Source: CAD feature listing. Evaluate the final solid. Frame: model axes, mm. Give positions to 0.01 mm unless a question says otherwise; leave off trailing zeros. Write each loop counter-clockwise with the first axis right and the second up, starting at its lowest first coordinate (ties: lowest second). Pieces come first, ordered by that corner, then holes. Notation, with made-up numbers: M -16,0 L 17,0 A25 cw 17,16 Z; hole C 37,-6 d9. An arc over 180 degrees is marked long. Use CSV: the item, a comma, the result in double quotes. Start each with the question number.
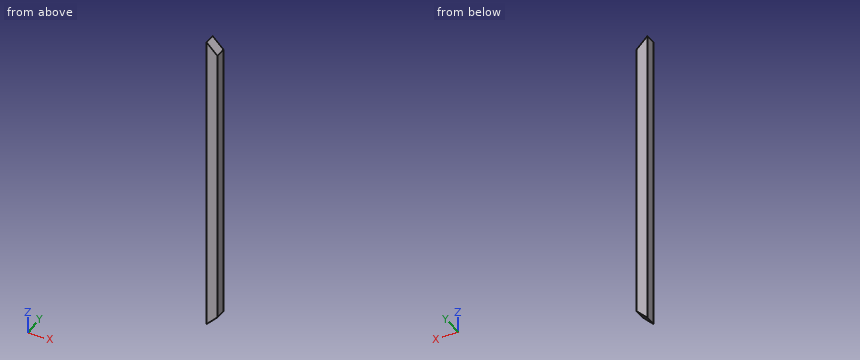
from build123d import *

# Parameters (mm, degrees)
F0_W     = 38.1
F0_H     = 38.1
F1_DEPTH = 1066.8
F3_DEPTH = 38.1
F4_DEPTH = 38.1


with BuildPart() as f1:
    # F0 (on Top) → F1 (new body)
    with BuildSketch(Plane.XY):
        Rectangle(F0_W, F0_H)
    extrude(amount=F1_DEPTH)

    # F2 (on face) → F3 (cut)
    with BuildSketch(Plane.XZ.offset(19.05)):
        Polygon((19.05, 1066.8), (-19.05, 1066.8), (19.05, 1028.7), align=None)
    extrude(amount=-F3_DEPTH, mode=Mode.SUBTRACT)

    # F2 (on face) → F4 (cut)
    with BuildSketch(Plane.XZ.offset(19.05)):
        Polygon((19.05, 38.1), (-19.05, 0), (19.05, 0), align=None)
    extrude(amount=-F4_DEPTH, mode=Mode.SUBTRACT)


solid = f1.part
Item 1: Material intervals for probe 1 along Z at (x, y) = (12, 7.5); probe 2 along Z at (x, y) = (-10, 10), sorted ascending.
Item 2: Section B-B (y = 1). Return the cut outline in (x, z), plus the area to 3 significant figures.
Item 3: Contact query for flat-ended pins moving along their axis: pin 1 Ø2 at (x, y) = (5.5, -12) entering from -Z; pin 2 Ø1.5 at (x, y) = (12.5, 12.5) entering from +Z; pin 3 Ø1.5 at (x, y) = (-1.5, -11.5) entering from -Z. Output: stop coordinate, or through.
Item 4: Section A-A (x = 3). Return the cut outline in (y, z).
Output values:
1,probe 1,"z = 31.05 to 1035.75"
1,probe 2,"z = 9.05 to 1057.75"
2,outline,"M -19.05,0 L 19.05,38.1 L 19.05,1028.7 L -19.05,1066.8 Z"
2,area,"39,200 mm2"
3,pin 1,"stops at z = 23.55"
3,pin 2,"stops at z = 1036"
3,pin 3,"stops at z = 16.8"
4,outline,"M -19.05,22.05 L 19.05,22.05 L 19.05,1044.75 L -19.05,1044.75 Z"
